Geometry: final body of the model. Coordinates: model frame, mm. A direction names the side the tool comes from. Coordinates: 2 decimals unless noted, no trailing zeros. Loops run counter-clockwise (first coordinate to the right, second up) from the corner with the lowest first, then second, coordinate; pieces in that order, holes last. Notation, with made-up numbers: (-24, -4.75) - (-4, -4.75) arc R26 ccw to (-4, 20.25) - close; hole circle Ø8 at (75, -23). An arc over 180 degrees is marked (long way). Answer in a Markdown table with one row per item.
from build123d import *

# Parameters (mm, degrees)
EXTRUDE_1_DEPTH           = 110
CUT_EXTRUDE_4_DEPTH       = 134.373777696
SKETCH_7_W                = 16.60831278
SKETCH_7_H                = 38.473598513
CUT_EXTRUDE_14_DEPTH      = 134.373777696
SKETCH_8_W                = 5
SKETCH_8_H                = 30.968526609
EXTRUDE_2_DEPTH           = 110
SKETCH_10_W               = 5
SKETCH_10_H               = 26
EXTRUDE_4_DEPTH           = 110
SKETCH_16_W               = 45
SKETCH_16_H               = 4
EXTRUDE_7_DEPTH           = 110
SKETCH_18_W               = 113.67218818
SKETCH_18_H               = 61.649849458
CUT_EXTRUDE_18_DEPTH      = 137.586229955
SKETCH_19_R               = 2.1
SKETCH_19_R_2             = 2
CUT_EXTRUDE_19_DEPTH      = 143.431323365
SKETCH_22_W               = 25
SKETCH_22_H               = 3
EXTRUDE_10_DEPTH          = 50
SKETCH_23_R               = 2
CUT_EXTRUDE_24_DEPTH      = 10
CUT_EXTRUDE_25_DEPTH      = 138.145152867
CUT_EXTRUDE_25_DEPTH_BACK = 138.145152867
SKETCH_24_W               = 94.85705968
SKETCH_24_H               = 31.336652995
SKETCH_24_W_2             = 96.91469655
SKETCH_24_H_2             = 33.70168341
SKETCH_26_W               = 42.056158723
SKETCH_26_H               = 66.577758737
CUT_EXTRUDE_26_DEPTH      = 85.230722286
EXTRUDE_11_DEPTH          = 5
SKETCH_28_R               = 2
SKETCH_28_W               = 19
SKETCH_28_H               = 27
CUT_EXTRUDE_27_DEPTH      = 109.719377855
EXTRUDE_13_DEPTH          = 5
EXTRUDE_14_DEPTH          = 25.02681365
EXTRUDE_15_DEPTH          = 25.02681365
CHAMFER_1_SIZE            = 4
CHAMFER_2_SIZE            = 3
CUT_EXTRUDE_28_DEPTH      = 2.5
CHAMFER_3_SIZE            = 2
CHAMFER_4_SIZE            = 2


with BuildPart() as part:
    # Эскиз1 → Бобышка-Вытянуть1 (new body)
    with BuildSketch(Plane(origin=(0, 0, 0), x_dir=(1, 0, 0), z_dir=(0, 1, 0))):
        Polygon((-66.825757576, 34.969739794), (-66.825757576, 29.969739794), (-63.825757576, 29.969739794), (-63.825757576, 31.969739794), (-38.825757576, 31.969739794), (-38.825757576, 6.969739794), (-63.825757576, 6.969739794), (-63.825757576, 8.969739794), (-66.825757576, 8.969739794), (-66.825757576, 3.969739794), (-22.123470102, 3.969739794), (-36.579007505, 34.969739794), align=None)
    extrude(amount=EXTRUDE_1_DEPTH)

    # Эскиз3 → Вырез-Вытянуть4 (cut, through all)
    with BuildSketch(Plane.XZ):
        Polygon((-66.825757576, -3.969739794), (-65.325757576, -8.969739794), (-66.825757576, -8.969739794), align=None)
        Polygon((-66.825757576, -29.969739794), (-66.825757576, -34.969739794), (-65.325757576, -29.969739794), align=None)
    extrude(amount=-CUT_EXTRUDE_4_DEPTH, mode=Mode.SUBTRACT)

    # Эскиз7 → Вырез-Вытянуть14 (cut, through all)
    with BuildSketch(Plane(origin=(0, 0, 0), x_dir=(-1, 0, 0), z_dir=(0, -1, 0))):
        with Locations((27.703474463, 20.539743139)):
            Rectangle(SKETCH_7_W, SKETCH_7_H)
    extrude(amount=-CUT_EXTRUDE_14_DEPTH, mode=Mode.SUBTRACT)

    # Эскиз8 → Бобышка-Вытянуть2 (add)
    with BuildSketch(Plane(origin=(0, 0, 0), x_dir=(-1, 0, 0), z_dir=(0, -1, 0))):
        with Locations((36.298943925, 19.454003098)):
            Rectangle(SKETCH_8_W, SKETCH_8_H)
    extrude(amount=-EXTRUDE_2_DEPTH)

    # Эскиз10 → Бобышка-Вытянуть4 (add)
    with BuildSketch(Plane.XZ):
        with Locations((-36.298943925, 9.030260206)):
            Rectangle(SKETCH_10_W, SKETCH_10_H)
    extrude(amount=-EXTRUDE_4_DEPTH)

    # Эскиз16 → Бобышка-Вытянуть7 (add, through all)
    with BuildSketch(Plane(origin=(0, 110, 0), x_dir=(1, 0, 0), z_dir=(0, 1, 0))):
        with Locations((-16.298943925, -24.030260206)):
            Rectangle(SKETCH_16_W, SKETCH_16_H)
    extrude(amount=-EXTRUDE_7_DEPTH)

    # Эскиз18 → Вырез-Вытянуть18 (cut, through all)
    with BuildSketch(Plane(origin=(6.201056075, 0, 0), x_dir=(0, 0, -1), z_dir=(1, 0, 0))):
        with Locations((3.709673157, 29.175075271)):
            Rectangle(SKETCH_18_W, SKETCH_18_H)
    extrude(amount=-CUT_EXTRUDE_18_DEPTH, mode=Mode.SUBTRACT)

    # Эскиз19 → Вырез-Вытянуть19 (cut, through all)
    with BuildSketch(Plane(origin=(0, 0, -34.969739794), x_dir=(-1, 0, 0), z_dir=(0, 0, -1))):
        with Locations((51.70238254, 85)):
            Circle(SKETCH_19_R)
        with Locations((3.798943925, 85)):
            Circle(SKETCH_19_R_2)
    extrude(amount=-CUT_EXTRUDE_19_DEPTH, mode=Mode.SUBTRACT)

    # Эскиз22 → Бобышка-Вытянуть10 (add)
    with BuildSketch(Plane.XZ.offset(-60)):
        with Locations((-21.298943925, -30.469739794)):
            Rectangle(SKETCH_22_W, SKETCH_22_H)
    extrude(amount=-EXTRUDE_10_DEPTH)

    # Эскиз23 → Вырез-Вытянуть24 (cut)
    with BuildSketch(Plane(origin=(0, 0, -31.969739794), x_dir=(-1, 0, 0), z_dir=(0, 0, -1))):
        with Locations((21.298943925, 85)):
            Circle(SKETCH_23_R)
    extrude(amount=-CUT_EXTRUDE_24_DEPTH, mode=Mode.SUBTRACT)

    # Эскиз24 → Вырез-Вытянуть25 (cut, two sides: drawn at the far end of the back side and taken through both)
    with BuildSketch(Plane(origin=(-62.400623407, 0, -18.720187022), x_dir=(-0.2873478855663458, 0, 0.9578262852211513), z_dir=(-0.9578262852211514, 0, -0.2873478855663458)).offset(-CUT_EXTRUDE_25_DEPTH_BACK)):
        with Locations((8.655390038, 113.168326498)):
            Rectangle(SKETCH_24_W, SKETCH_24_H)
        with Locations((7.626571603, 55.649158295)):
            Rectangle(SKETCH_24_W_2, SKETCH_24_H_2)
    extrude(amount=CUT_EXTRUDE_25_DEPTH + CUT_EXTRUDE_25_DEPTH_BACK, mode=Mode.SUBTRACT)

    # Эскиз26 → Вырез-Вытянуть26 (cut, through all)
    with BuildSketch(Plane.XZ.offset(-60)):
        with Locations((-12.770864564, -1.649387034)):
            Rectangle(SKETCH_26_W, SKETCH_26_H)
    extrude(amount=-CUT_EXTRUDE_26_DEPTH, mode=Mode.SUBTRACT)

    # Эскиз27 → Бобышка-Вытянуть11 (add)
    with BuildSketch(Plane(origin=(-33.798943925, 0, 0), x_dir=(0, 0, -1), z_dir=(1, 0, 0))):
        Polygon((-26.030260206, 72.5), (4.449739794, 72.5), (4.449739794, 42.7), (-26.030260206, 35.043953179), align=None)
    extrude(amount=-EXTRUDE_11_DEPTH)

    # Эскиз28 → Вырез-Вытянуть27 (cut, through all)
    with BuildSketch(Plane(origin=(-33.798943925, 0, 0), x_dir=(0, 0, -1), z_dir=(1, 0, 0))):
        with Locations((-10.603567011, 89.464970071)):
            Circle(SKETCH_28_R)
        with Locations((-10.790260206, 48.464970071)):
            Circle(SKETCH_28_R)
        with Locations((-10.790260206, 68.964970071)):
            Rectangle(SKETCH_28_W, SKETCH_28_H)
    extrude(amount=-CUT_EXTRUDE_27_DEPTH, mode=Mode.SUBTRACT)

    # Эскиз29 → Бобышка-Вытянуть13 (add)
    with BuildSketch(Plane(origin=(-33.798943925, 0, 0), x_dir=(0, 0, -1), z_dir=(1, 0, 0))):
        Polygon((-7.290260206, 82.464970071), (-1.290260206, 82.464970071), (-1.290260206, 76.964970071), align=None)
        Polygon((-1.290260206, 60.964970071), (-7.290260206, 55.464970071), (-1.290260206, 55.464970071), align=None)
    extrude(amount=-EXTRUDE_13_DEPTH)

    # Эскиз30 → Бобышка-Вытянуть14 (add)
    with BuildSketch(Plane.ZY.offset(38.798943925)):
        Polygon((-4.449739794, 42.7), (-4.449739794, 97.5), (-1.449739794, 97.5), (-1.449739794, 45.039643715), (26.030260206, 38.137144809), (26.030260206, 35.043953179), align=None)
    extrude(amount=EXTRUDE_14_DEPTH)

    # Эскиз32 → Бобышка-Вытянуть15 (add)
    with BuildSketch(Plane.ZY.offset(38.798943925)):
        Polygon((-1.449739794, 97.5), (26.030260206, 97.5), (26.030260206, 38.137144809), (24.030260206, 38.639510086), (24.030260206, 95.5), (-1.449739794, 95.5), align=None)
    extrude(amount=EXTRUDE_15_DEPTH)

    # Фаска1
    chamfer_1_edges = [part.edges().sort_by_distance(p)[0] for p in [
        (-48.81235075, 97.5, 26.030260206),
    ]]
    chamfer(chamfer_1_edges, length=CHAMFER_1_SIZE - 0.0001)  # a hair under: the kernel refuses the full size

    # Фаска2
    chamfer_2_edges = [part.edges().sort_by_distance(p)[0] for p in [
        (-51.31235075, 95.5, 24.030260206),
    ]]
    chamfer(chamfer_2_edges, length=CHAMFER_2_SIZE)

    # Эскиз33 → Вырез-Вытянуть28 (cut)
    with BuildSketch(Plane.ZY.offset(38.798943925)):
        Polygon((10.603567011, 93.506421955), (7.103567011, 91.485696013), (7.103567011, 87.444244129), (10.603567011, 85.423518186), (14.103567011, 87.444244129), (14.103567011, 91.485696013), align=None)
        Polygon((10.790260206, 52.506421955), (7.290260206, 50.485696013), (7.290260206, 46.444244129), (10.790260206, 44.423518186), (14.290260206, 46.444244129), (14.290260206, 50.485696013), align=None)
    extrude(amount=-CUT_EXTRUDE_28_DEPTH, mode=Mode.SUBTRACT)

    # Фаска3
    chamfer_3_edges = [part.edges().sort_by_distance(p)[0] for p in [
        (-33.798943925, 72.5, -19.694003099),
        (-33.798943925, 57.6, -4.449739794),
    ]]
    chamfer(chamfer_3_edges, length=CHAMFER_3_SIZE)

    # Фаска4
    chamfer_4_edges = [part.edges().sort_by_distance(p)[0] for p in [
        (-33.798943925, 38.620793951, 11.790260206),
    ]]
    chamfer(chamfer_4_edges, length=CHAMFER_4_SIZE)


solid = part.part
(1) Cut plane C-C on y = 54. Output: boundary loops of the cut face in (x, z).
Verdict:
| item | result |
|---|---|
| outline | (-63.83, -4.45) - (-35.8, -4.45) - (-33.8, -2.45) - (-33.8, 26.03) - (-63.83, 26.03) - (-63.83, 24.03) - (-38.8, 24.03) - (-38.8, -1.45) - (-63.83, -1.45) - close |
(2) Pull-direction query (Z, two-part tool) for faces 1 (the face through (-51.137, 41.884, 11.112)), 2 (the face through (-34.8, 39.9, 10.8)), 3 (the face through (-38.6, 72.5, -17.2)); classes: pulls with the +Z half, pulls with the -Z half, needs draft (parallel to the pull), parting line crosses it, or undercut.
Verdict:
| item | result |
|---|---|
| face 1 | undercut |
| face 2 | pulls with the -Z half |
| face 3 | needs draft |
(3) First-contact query: pin 1 Ø15 at (y, z) = (59, 9) entering from -X; pin 2 Ø6.5 at (x, z) = (-49.5, 5.5) entering from -Y; pin 3 Ø1.6 at (x, y) = (-65, 90) entering from +Z. Flat tips, straight axial feed; report the tip coordinate or a pass-through.
Verdict:
| item | result |
|---|---|
| pin 1 | stops at x = -38.8 |
| pin 2 | stops at y = 39.38 |
| pin 3 | stops at z = -3.97 |
(4) Cut plane A-A on x = -57. Output: boundary loops of the cut face in (y, z), then the cut area to 3 significant figures.
Verdict:
| item | result |
|---|---|
| outline | (35.04, 26.03) - (42.7, -4.45) - (72.5, -4.45) - (72.5, -6.97) - (97.5, -6.97) - (97.5, 22.03) - (93.5, 26.03) - close; (72.5, -34.97) - (97.5, -34.97) - (97.5, -31.97) - (72.5, -31.97) - close; hole (38.64, 24.03) - (45.04, -1.45) - (95.5, -1.45) - (95.5, 21.03) - (92.5, 24.03) - close |
| area | 554 mm² |
(5) Cut plane B-B on z = 15.5. Output: boundary loops of the cut face in (x, y), then the cut area to 3 significant figures.
Verdict:
| item | result |
|---|---|
| outline | (-63.83, 37.69) - (-35.8, 37.69) - (-33.8, 39.75) - (-33.8, 55.46) - (-38.8, 55.46) - (-38.8, 40.78) - (-63.83, 40.78) - close; (-63.83, 95.5) - (-38.8, 95.5) - (-38.8, 82.46) - (-33.8, 82.46) - (-33.8, 97.5) - (-63.83, 97.5) - close |
| area | 289 mm² |
(6) Cut plane D-D on z = -25. Output: boundary loops of the cut face in (x, y), then the cut area to 3 significant figures.
Verdict:
| item | result |
|---|---|
| outline | (-38.83, 72.5) - (-35.8, 72.5) - (-33.8, 74.5) - (-33.8, 97.5) - (-38.83, 97.5) - close |
| area | 124 mm² |
(7) Ray query, probe 1 along Z at (x, y) = (-55, 82.5); probe 2 along Z at (x, y) = (-57.5, 63); probe 3 along Z at (x, y) = (-64, 73.5). Return the intervals inside material, ascending.
Verdict:
| item | result |
|---|---|
| probe 1 | z = -34.97 to -31.97, -6.97 to -1.45, 24.03 to 26.03 |
| probe 2 | z = -4.45 to -1.45, 24.03 to 26.03 |
| probe 3 | z = -34.97 to -29.97, -8.97 to -3.97 |
(8) Access query for faces 4 (the face through (-36, 82.465, 14)), 5 (the face through (-51, 65, 24.03)), 6 (the face through (-65, 85, -29.97)), 7 (the face through (-34.8, 73.5, -18.9)). Directions: +Z, -Z, +X, -X, +Y, -Y. A direction counts if a zero-diameter tool reaches every point of the face in a straight line with its end or side. Return the directions, or none.
Verdict:
| item | result |
|---|---|
| face 4 | +X, -X |
| face 5 | -X |
| face 6 | -X, +Y, -Y |
| face 7 | -Z, +X, -Y |
